For this review, take the finished solid that the model builds, in its own axes (mm). A direction names the side the tool comes from. Round coordinates to 2 decimals unless told otherwise and drop trailing zeros. Order: outer loops, then holes, each group sorted by start corner. A loop starts at its lowest first (then second) coordinate and runs counter-clockwise, first axis right, second up. Notation, with made-up numbers: (41.25, 6.5) -> (45.25, 6.5) arc R25 cw to (45.25, 39.5) -> close; hole circle Ø6 at (-11, 16). An arc over 180 degrees is marked (long way). Answer in a Markdown table with one row per item.
```python
from build123d import *

# Parameters (mm, degrees)
SKETCH1_R           = 1.65
BOSS_EXTRUDE1_DEPTH = 8.5
SKETCH2_R           = 2.1
BOSS_EXTRUDE2_DEPTH = 3.175
FILLET1_R           = 2
CUT_EXTRUDE1_START  = -10
CUT_EXTRUDE1_DEPTH  = 10


with BuildPart() as part:
    # Sketch1 → Boss-Extrude1 (new body)
    with BuildSketch(Plane(origin=(0, 0, 0), x_dir=(0, 0, -1), z_dir=(1, 0, 0))):
        with BuildLine():
            Line((-13, -6), (13, -6))
            ThreePointArc((13, -6), (14.414213562, -5.414213562), (15, -4))
            Line((15, -4), (15, 4))
            ThreePointArc((15, 4), (14.414213562, 5.414213562), (13, 6))
            Line((13, 6), (-13, 6))
            ThreePointArc((-13, 6), (-14.414213562, 5.414213562), (-15, 4))
            Line((-15, 4), (-15, -4))
            ThreePointArc((-15, -4), (-14.414213562, -5.414213562), (-13, -6))
        make_face()
        with Locations((-11.8, 0)):
            Circle(SKETCH1_R, mode=Mode.SUBTRACT)
        with Locations((11.8, 0)):
            Circle(SKETCH1_R, mode=Mode.SUBTRACT)
    extrude(amount=BOSS_EXTRUDE1_DEPTH)

    # Sketch2 → Boss-Extrude2 (add, symmetric)
    with BuildSketch(Plane.XY):
        with BuildLine():
            Line((25.918129472, 25.580456988), (3.805255429, -6))
            Line((3.805255429, -6), (0, -3.335531464))
            Line((0, -3.335531464), (0, 6))
            Line((0, 6), (17.726609029, 31.316221351))
            ThreePointArc((17.726609029, 31.316221351), (19.017616762, 32.138683985), (20.51206599, 31.807372567))
            Line((20.51206599, 31.807372567), (25.426978256, 28.365913949))
            ThreePointArc((25.426978256, 28.365913949), (26.249440889, 27.074906216), (25.918129472, 25.580456988))
        make_face()
        with Locations((20.675216378, 26.810035081)):
            Circle(SKETCH2_R, mode=Mode.SUBTRACT)
        with Locations((16.883876134, 21.395440068)):
            Circle(SKETCH2_R, mode=Mode.SUBTRACT)
        with Locations((13.092535889, 15.980845055)):
            Circle(SKETCH2_R, mode=Mode.SUBTRACT)
        with Locations((9.301195645, 10.566250043)):
            Circle(SKETCH2_R, mode=Mode.SUBTRACT)
    extrude(amount=BOSS_EXTRUDE2_DEPTH, both=True)

    # Fillet1
    fillet1_edges = [part.edges().sort_by_distance(p)[0] for p in [
        (8.5, 0.704790101, 0),
    ]]
    fillet(fillet1_edges, radius=FILLET1_R)

    # Sketch4 → Cut-Extrude1 (cut)
    with BuildSketch(Plane(origin=(8.5, 0, 0), x_dir=(0, 0, -1), z_dir=(1, 0, 0)).offset(CUT_EXTRUDE1_START)):
        with BuildLine():
            Line((-15, 0), (-15, -4))
            ThreePointArc((-15, -4), (-14.414213562, -5.414213562), (-13, -6))
            Line((-13, -6), (13, -6))
            ThreePointArc((13, -6), (14.414213562, -5.414213562), (15, -4))
            Line((15, -4), (15, 0))
            ThreePointArc((15, 0), (13.501034406, -2.710439438), (10.408448782, -2.881594213))
            ThreePointArc((10.408448782, -2.881594213), (0, -0.5), (-10.408448782, -2.881594213))
            ThreePointArc((-10.408448782, -2.881594213), (-13.501034406, -2.710439438), (-15, 0))
        make_face()
    extrude(amount=CUT_EXTRUDE1_DEPTH, mode=Mode.SUBTRACT)


solid = part.part
```
Q1. Take a section at C-C, the plane x = 3. Write out the cut boundary in (y, z) (3 decimals).
Answer key:
| item | result |
|---|---|
| outline | (-2.882, -10.408) arc R3.2 ccw to (0, -15) -> (4, -15) arc R2 ccw to (6, -13) -> (6, -3.175) -> (10.284, -3.175) -> (10.284, 3.175) -> (6, 3.175) -> (6, 13) arc R2 ccw to (4, 15) -> (0, 15) arc R3.2 ccw to (-2.882, 10.408) arc R23.935 cw to start; hole circle Ø3.3 at (0, -11.8); hole circle Ø3.3 at (0, 11.8) |
Q2. The part is to be moulded in two halves that separate along Z. For faces 1 (the face through (4, 2, 15)), 2 (the face through (4.19, 5.4, -14.43)), 3 (the face through (4.19, -0.632, -13.324)), 4 (the face through (4, 6, 8)), say which applies: +Z half, -Z half, draft (parallel to the pull), parting line (faces both ways), or undercut.
Answer key:
| item | result |
|---|---|
| face 1 | +Z half |
| face 2 | -Z half |
| face 3 | undercut |
| face 4 | draft |
Q3. Tool access review of faces 5 (the face through (18.01, 23.17, -0.04)), 6 (the face through (4, 6, -8)): name each direction out of +Z, -Z, +X, -X, +Y, -Y from which nothing blocks a thin tool from reaching the whole face with its end or side.
Answer key:
| item | result |
|---|---|
| face 5 | +Z, -Z |
| face 6 | -Z, +X, -X, +Y |
Q4. Take a section at B-B, the plane x = 9.5. Write out the cut boundary in (y, z) (3 decimals).
Answer key:
| item | result |
|---|---|
| outline | (2.133, -3.175) -> (8.476, -3.175) -> (8.476, 3.175) -> (2.133, 3.175) -> close; (12.657, -3.175) -> (19.567, -3.175) -> (19.567, 3.175) -> (12.657, 3.175) -> close |
Q5. Clearance check with flat-ended pins moving along their axes: pin 1 Ø7 at (x, z) = (5.5, 8.5) entering from +Y; pin 2 Ø3.5 at (x, y) = (16.88, 21.4) entering from -Z; pin 3 Ø1.5 at (x, z) = (14.5, -0.5) entering from +Y; pin 4 Ø5.5 at (y, z) = (0, 11.8) entering from +X. State where each tip first meets the part, or that it passes through.
Answer key:
| item | result |
|---|---|
| pin 1 | stops at y = 6 |
| pin 2 | passes through |
| pin 3 | stops at y = 27.78 |
| pin 4 | stops at x = 8.5 |
Q6. Take a section at A-A, the plane z = -11.8. Write out the cut boundary in (x, y).
Answer key:
| item | result |
|---|---|
| outline | (0, -3.2) -> (8.5, -3.2) -> (8.5, -1.65) -> (0, -1.65) -> close; (0, 1.65) -> (8.5, 1.65) -> (8.5, 6) -> (0, 6) -> close |
Q7. Take a section at D-D, the plane z = 6.25. Write out the cut boundary in (x, y).
Answer key:
| item | result |
|---|---|
| outline | (0, -1.33) -> (8.5, -1.33) -> (8.5, 6) -> (0, 6) -> close |
Q8. To check wall thickness, follow probe 1 along Y at (x, z) = (6, 11.8); probe 2 along Z at (x, y) = (20.5, 20) (3 decimals); probe 3 along Y at (x, z) = (5.5, -10.5). State the ranges of each line that lie inside material, in increasing order.
Answer key:
| item | result |
|---|---|
| probe 1 | y = -3.2 to -1.65, 1.65 to 6 |
| probe 2 | z = -3.175 to 3.175 |
| probe 3 | y = -2.92 to -1.02, 1.02 to 6 |
